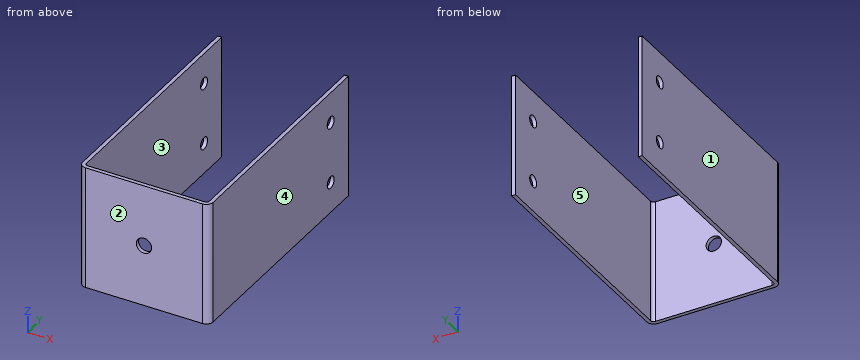
from build123d import *

# Parameters (mm, degrees)
SKETCH9_W                    = 50.8
SKETCH9_H                    = 1.5875
BASE_FLANGE1_DEPTH           = 50.8
EDGE_FLANGE1_STRIP_W         = 8.89
EDGE_FLANGE1_STRIP_H         = 1.5875
EDGE_FLANGE1_STRIP_CUT_DEPTH = 50.8
EDGE_FLANGE1_DEPTH           = 50.8
EDGE_FLANGE2_STRIP_W         = 8.89
EDGE_FLANGE2_STRIP_H         = 1.5875
EDGE_FLANGE2_STRIP_CUT_DEPTH = 50.8
EDGE_FLANGE2_DEPTH           = 50.8
SKETCH20_R                   = 2.4892
CUT_EXTRUDE1_DEPTH           = 124.263641262
CUT_EXTRUDE2_DEPTH           = 124.855948312
CUT_EXTRUDE2_DEPTH_BACK      = 124.855948312
SKETCH21_R                   = 3.175


# Sheet-metal steps are written as plain solids
with BuildPart() as part:
    # Sketch9 → Base-Flange1 (new body)
    with BuildSketch(Plane.XY):
        with Locations((25.4, -0.79375)):
            Rectangle(SKETCH9_W, SKETCH9_H)
    extrude(amount=BASE_FLANGE1_DEPTH)

    # Edge-Flange1 strip (across the edge) → Edge-Flange1 strip cut (cut)
    with BuildSketch(Plane.XY):
        with Locations((-3.175, -0.79375)):
            Rectangle(EDGE_FLANGE1_STRIP_W, EDGE_FLANGE1_STRIP_H)
    extrude(amount=EDGE_FLANGE1_STRIP_CUT_DEPTH, mode=Mode.SUBTRACT)

    # Edge-Flange1 section (across the edge) → Edge-Flange1 (add)
    with BuildSketch(Plane.XY):
        with BuildLine():
            Line((-1.5875, 1.27), (-1.5875, 98.4885))
            Line((-1.5875, 98.4885), (0, 98.4885))
            Line((0, 98.4885), (0, 1.27))
            ThreePointArc((0, 1.27), (0.371974388, 0.371974388), (1.27, 0))
            Line((1.27, 0), (1.27, -1.5875))
            ThreePointArc((1.27, -1.5875), (-0.750557627, -0.750557627), (-1.5875, 1.27))
        make_face()
    extrude(amount=EDGE_FLANGE1_DEPTH)

    # Edge-Flange2 strip (across the edge) → Edge-Flange2 strip cut (cut)
    with BuildSketch(Plane(origin=(50.8, 0, 50.8), x_dir=(-1, 0, 0), z_dir=(0, 0, -1))):
        with Locations((-3.175, -0.79375)):
            Rectangle(EDGE_FLANGE2_STRIP_W, EDGE_FLANGE2_STRIP_H)
    extrude(amount=EDGE_FLANGE2_STRIP_CUT_DEPTH, mode=Mode.SUBTRACT)

    # Edge-Flange2 section (across the edge) → Edge-Flange2 (add)
    with BuildSketch(Plane(origin=(50.8, 0, 50.8), x_dir=(-1, 0, 0), z_dir=(0, 0, -1))):
        with BuildLine():
            Line((-1.5875, 1.27), (-1.5875, 98.4885))
            Line((-1.5875, 98.4885), (0, 98.4885))
            Line((0, 98.4885), (0, 1.27))
            ThreePointArc((0, 1.27), (0.371974388, 0.371974388), (1.27, 0))
            Line((1.27, 0), (1.27, -1.5875))
            ThreePointArc((1.27, -1.5875), (-0.750557627, -0.750557627), (-1.5875, 1.27))
        make_face()
    extrude(amount=EDGE_FLANGE2_DEPTH)

    # Sketch20 → Cut-Extrude1 (cut, through all)
    with BuildSketch(Plane(origin=(52.3875, 0, 0), x_dir=(0, 0, -1), z_dir=(1, 0, 0))):
        with Locations(Location((-38.1, 85.7885, 0), (0, 0, 90))):
            Circle(SKETCH20_R)
        with Locations(Location((-12.7, 85.7885, 0), (0, 0, 90))):
            Circle(SKETCH20_R)
    extrude(amount=-CUT_EXTRUDE1_DEPTH, mode=Mode.SUBTRACT)

    # Sketch21 → Cut-Extrude2 (cut, two sides: drawn at the far end of the back side and taken through both)
    with BuildSketch(Plane.XZ.offset(1.5875).offset(-CUT_EXTRUDE2_DEPTH_BACK)):
        with Locations(Location((25.4, 25.4, 0), (0, 0, 90))):
            Circle(SKETCH21_R)
    extrude(amount=CUT_EXTRUDE2_DEPTH + CUT_EXTRUDE2_DEPTH_BACK, mode=Mode.SUBTRACT)


solid = part.part
Design review of the part built by this model. Coordinates are the model's own, in mm. Face numbers are marked on the shaded views. A direction names the side the tool comes from. Round coordinates to 2 decimals unless told otherwise and drop trailing zeros. Loops run counter-clockwise (first coordinate to the right, second up) from the corner with the lowest first, then second, coordinate; pieces in that order, holes last. Notation, with made-up numbers: (31.25, 58.5) - (73.25, 58.5) arc R16 ccw to (73.25, 62.5) - close; hole circle Ø10 at (-11.75, 24). An arc over 180 degrees is marked (long way). One line per item, written item: value. Start each with the question number.
1) Consider section A-A on z = 25.4. Give the boundary of the cut face in (x, y) (1 decimal).
2) To check wall thickness, follow L1, parallel to X at y = 17.5, z = 11; L2, parallel to Y at x = 10.5, z = 5; L3, parallel to X at y = -1, z = 25.4 (3 decimals). State the ranges of each line that lie inside material, in increasing order. Write a range as from..to.
3) Consider section B-B on x = 25.4. Give the boundary of the cut face in (y, z) (1 decimal).
4) Draft analysis for pull direction X (two halves, no side actions). For the marked faces 1, 2 and 3, state which applies: +X half, -X half, draft (parallel to the pull), parting line (faces both ways), or undercut.
5) Insertion check: pin 1 Ø14.5 at (x, z) = (35.5, 27.5) entering from +Y. The pin has a flat end and moves straight along its axis. Give the tip position at first contact, or say it passes through.
6) Consider section D-D on y = 8.5. Give the boundary of the cut face in (x, z), then the cut area to 3 significant figures.
7) Consider section C-C on z = 12.7. Give the boundary of the cut face in (x, y) (1 decimal).
8) For the marked faces 4 and 5, list the 3-axis set-ups (+Z, -Z, +X, -X, +Y, -Y) from which the entire face can be reached by the end or side of a thin tool; tool diameter is ignored.
Reported:
1. outline: (-1.6, 1.3) arc R2.9 ccw to (1.3, -1.6) - (22.2, -1.6) - (22.2, 0) - (1.3, 0) arc R1.3 cw to (0, 1.3) - (0, 98.5) - (-1.6, 98.5) - close; (28.6, -1.6) - (49.5, -1.6) arc R2.9 ccw to (52.4, 1.3) - (52.4, 98.5) - (50.8, 98.5) - (50.8, 1.3) arc R1.3 cw to (49.5, 0) - (28.6, 0) - close
2. L1: x = -1.59..0, 50.8..52.39
2. L2: y = -1.59..0
2. L3: x = -0.466..22.225, 28.575..51.266
3. outline: (-1.6, 0) - (0, 0) - (0, 22.2) - (-1.6, 22.2) - close; (-1.6, 28.6) - (0, 28.6) - (0, 50.8) - (-1.6, 50.8) - close
4. face 1: -X half
4. face 2: draft
4. face 3: undercut
5. pin 1: stops at y = 0
6. outline: (-1.59, 0) - (0, 0) - (0, 50.8) - (-1.59, 50.8) - close; (50.8, 0) - (52.39, 0) - (52.39, 50.8) - (50.8, 50.8) - close
6. area: 161 mm^2
7. outline: (-1.6, 1.3) arc R2.9 ccw to (1.3, -1.6) - (49.5, -1.6) arc R2.9 ccw to (52.4, 1.3) - (52.4, 83.3) - (50.8, 83.3) - (50.8, 1.3) arc R1.3 cw to (49.5, 0) - (1.3, 0) arc R1.3 cw to (0, 1.3) - (0, 83.3) - (-1.6, 83.3) - close; (-1.6, 88.3) - (0, 88.3) - (0, 98.5) - (-1.6, 98.5) - close; (50.8, 88.3) - (52.4, 88.3) - (52.4, 98.5) - (50.8, 98.5) - close
8. face 4: +Z, -Z, +X, +Y, -Y
8. face 5: +Z, -Z, +Y
